For this review, use the dimensioned drawing (mm, ordinates from the lowest corner) and the shaded views. A direction names the side the tool comes from. Round coordinates to 2 decimals unless told otherwise and drop trailing zeros. Write each loop counter-clockwise with the first axis right and the second up, starting at its lowest first coordinate (ties: lowest second). Pieces come first, ordered by that corner, then holes. Notation, with made-up numbers: (82.5, 28.5) -> (108.5, 28.5) arc R27 cw to (108.5, 60.5) -> close; hole circle Ø7 at (17, -32). An arc over 180 degrees is marked (long way). Answer in a Markdown table with one row per item. Add a question column.
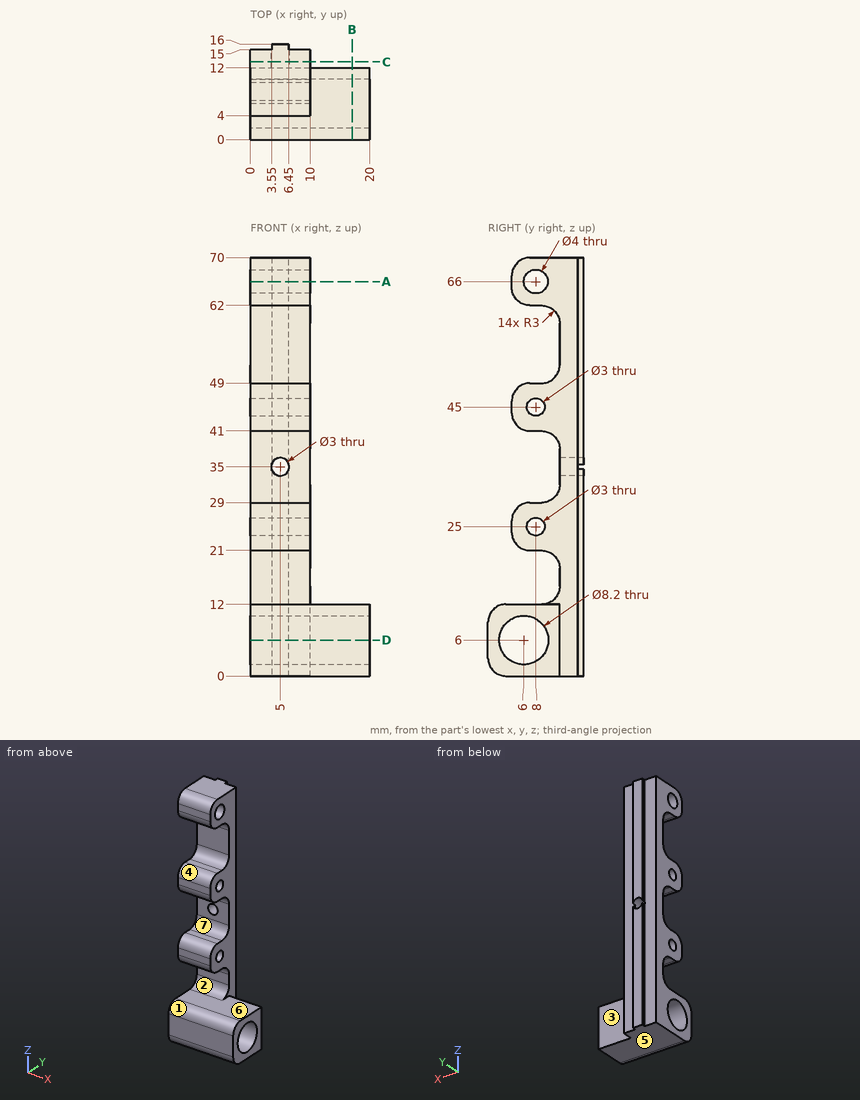
1. We need section C-C (y = 13). Write out the cut boundary in (x, z), plus the area to 3 significant figures.
2. We need section B-B (x = 17). Write out the cut boundary in (y, z), plus the area to 3 significant figures.
3. We need section A-A (z = 66). Write out the cut boundary in (x, y), plus the area to 3 significant figures.
4. Clearance check with flat-ended pins moving along their axes: pin 1 Ø12 at (x, z) = (17.5, 11.5) entering from +Y; pin 2 Ø3 at (x, y) = (15.5, 11) entering from +Z; pin 3 Ø3.5 at (y, z) = (9.5, 49) entering from +X; pin 4 Ø1.6 at (x, y) = (4, 8) entering from -Z. State where each tip first meets the part, or that it passes through.
5. We need section D-D (z = 6). Write out the cut boundary in (x, y), plus the area to 3 significant figures.
6. Tool access review of the marked faces 5, 6 and 7: name each direction out of +Z, -Z, +X, -X, +Y, -Y from which nothing blocks a thin tool from reaching the whole face with its end or side.
7. For L1, parallel to Y at x = 4, z = 25; L2, parallel to Z at x = 5, y = 15; L3, parallel to X at y = 13.25, z = 35, list the stretches that pass through material, from the lowest coordinate up. Write a range as [from, to].
8. The part is to be moulded in two halves that separate along Z. For the marked faces 1, 2, 3 and 4, say which applies: pulls with the +Z half, pulls with the -Z half, needs draft (parallel to the pull), parting line crosses it, or undercut.
Response:
| question | item | result |
|---|---|---|
| 1 | outline | (0, 0) -> (10, 0) -> (10, 70) -> (0, 70) -> close; hole circle Ø3 at (5, 35) |
| 1 | area | 693 mm2 |
| 2 | outline | (0, 3) arc R3 ccw to (3, 0) -> (12, 0) -> (12, 12) -> (3, 12) arc R3 ccw to (0, 9) -> close; hole circle Ø8.2 at (6, 6) |
| 2 | area | 87.3 mm2 |
| 3 | outline | (0, 4) -> (10, 4) -> (10, 6) -> (0, 6) -> close; (0, 10) -> (10, 10) -> (10, 15) -> (6.45, 15) -> (6.45, 16) -> (3.55, 16) -> (3.55, 15) -> (0, 15) -> close |
| 3 | area | 72.9 mm2 |
| 4 | pin 1 | y = 12 |
| 4 | pin 2 | z = 12 |
| 4 | pin 3 | x = 10 |
| 4 | pin 4 | z = 0 |
| 5 | outline | (0, 0) -> (20, 0) -> (20, 1.9) -> (0, 1.9) -> close; (0, 10.1) -> (20, 10.1) -> (20, 12) -> (10, 12) -> (10, 15) -> (6.45, 15) -> (6.45, 16) -> (3.55, 16) -> (3.55, 15) -> (0, 15) -> close |
| 5 | area | 109 mm2 |
| 6 | face 5 | -Z, +X, -X, +Y, -Y |
| 6 | face 6 | +X, -Y |
| 6 | face 7 | +X, -X, -Y |
| 7 | L1 | [4, 6.5], [9.5, 16] |
| 7 | L2 | [0, 33.5], [36.5, 70] |
| 7 | L3 | [0, 3.5], [6.5, 10] |
| 8 | face 1 | pulls with the +Z half |
| 8 | face 2 | undercut |
| 8 | face 3 | needs draft |
| 8 | face 4 | undercut |
